from build123d import *

# Parameters (mm, degrees)
MODEL_R                 = 17.5
MODEL_R_2               = 1.5
SALIENTE_EXTRUIR1_DEPTH = 3


with BuildPart() as part:
    # Model → Saliente-Extruir1 (new body)
    with BuildSketch(Plane.XY):
        with BuildLine():
            Line((119.290027295, 223.651688958), (119.290027295, 219.036053988))
            Line((119.290027295, 219.036053988), (123.790027295, 219.036053988))
            Line((123.790027295, 219.036053988), (123.790027295, 210.036053988))
            Line((123.790027295, 210.036053988), (119.290027295, 210.036053988))
            Line((119.290027295, 210.036053988), (119.290027295, 183.036053988))
            Line((119.290027295, 183.036053988), (141.790027295, 183.036053988))
            Line((141.790027295, 183.036053988), (141.790027295, 192.036053988))
            Line((141.790027295, 192.036053988), (150.790027295, 192.036053988))
            Line((150.790027295, 192.036053988), (150.790027295, 183.036053988))
            Line((150.790027295, 183.036053988), (173.290027295, 183.036053988))
            Line((173.290027295, 183.036053988), (173.290027295, 210.036053988))
            Line((173.290027295, 210.036053988), (168.790027295, 210.036053988))
            Line((168.790027295, 210.036053988), (168.790027295, 219.036053988))
            Line((168.790027295, 219.036053988), (173.290027295, 219.036053988))
            Line((173.290027295, 219.036053988), (173.290027295, 223.651688958))
            Line((173.290027295, 223.651688958), (166.290027295, 229.536053988))
            ThreePointArc((166.290027295, 229.536053988), (164.825561201, 233.071587894), (161.290027295, 234.536053988))
            Line((161.290027295, 234.536053988), (131.290027295, 234.536053988))
            ThreePointArc((131.290027295, 234.536053988), (127.754493389, 233.071587894), (126.290027295, 229.536053988))
            Line((126.290027295, 229.536053988), (119.290027295, 223.651688958))
        make_face()
        with Locations((146.290027295, 214.536053988)):
            Circle(MODEL_R, mode=Mode.SUBTRACT)
        with Locations((168.790027295, 223.536053988)):
            Circle(MODEL_R_2, mode=Mode.SUBTRACT)
        with Locations((161.290027295, 229.536053988)):
            Circle(MODEL_R_2, mode=Mode.SUBTRACT)
        with Locations((168.790027295, 187.536053988)):
            Circle(MODEL_R_2, mode=Mode.SUBTRACT)
        with Locations((161.290027295, 199.536053988)):
            Circle(MODEL_R_2, mode=Mode.SUBTRACT)
        with Locations((123.790027295, 223.536053988)):
            Circle(MODEL_R_2, mode=Mode.SUBTRACT)
        with Locations((131.290027295, 229.536053988)):
            Circle(MODEL_R_2, mode=Mode.SUBTRACT)
        with Locations((131.290027295, 199.536053988)):
            Circle(MODEL_R_2, mode=Mode.SUBTRACT)
        with Locations((123.790027295, 187.536053988)):
            Circle(MODEL_R_2, mode=Mode.SUBTRACT)
        with BuildLine():
            Line((122.290027295, 203.286053988), (122.290027295, 198.786053988))
            ThreePointArc((122.290027295, 198.786053988), (123.790027295, 197.286053988), (125.290027295, 198.786053988))
            Line((125.290027295, 198.786053988), (125.290027295, 203.286053988))
            ThreePointArc((125.290027295, 203.286053988), (123.790027295, 204.786053988), (122.290027295, 203.286053988))
        make_face(mode=Mode.SUBTRACT)
        with BuildLine():
            Line((167.290027295, 203.286053988), (167.290027295, 198.786053988))
            ThreePointArc((167.290027295, 198.786053988), (168.790027295, 197.286053988), (170.290027295, 198.786053988))
            Line((170.290027295, 198.786053988), (170.290027295, 203.286053988))
            ThreePointArc((170.290027295, 203.286053988), (168.790027295, 204.786053988), (167.290027295, 203.286053988))
        make_face(mode=Mode.SUBTRACT)
        with BuildLine():
            Line((162.040027295, 189.036053988), (157.540027295, 189.036053988))
            ThreePointArc((157.540027295, 189.036053988), (156.040027295, 187.536053988), (157.540027295, 186.036053988))
            Line((157.540027295, 186.036053988), (162.040027295, 186.036053988))
            ThreePointArc((162.040027295, 186.036053988), (163.540027295, 187.536053988), (162.040027295, 189.036053988))
        make_face(mode=Mode.SUBTRACT)
        with BuildLine():
            Line((135.040027295, 186.036053988), (130.540027295, 186.036053988))
            ThreePointArc((130.540027295, 186.036053988), (129.040027295, 187.536053988), (130.540027295, 189.036053988))
            Line((130.540027295, 189.036053988), (135.040027295, 189.036053988))
            ThreePointArc((135.040027295, 189.036053988), (136.540027295, 187.536053988), (135.040027295, 186.036053988))
        make_face(mode=Mode.SUBTRACT)
    extrude(amount=SALIENTE_EXTRUIR1_DEPTH)


solid = part.part
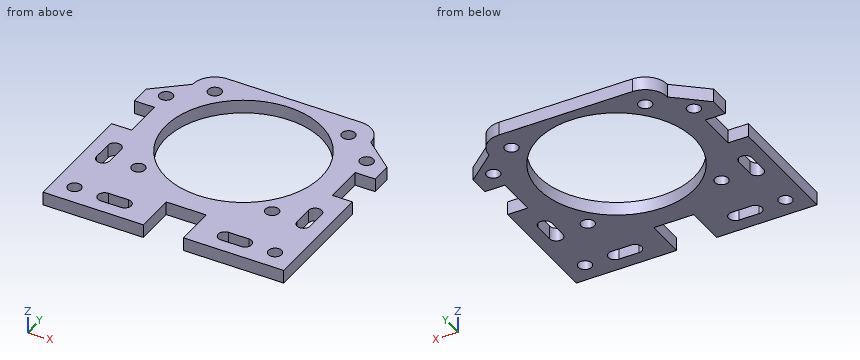
The listing builds one solid part. Answer for the finished solid, in the listing's coordinates (mm). Give positions to 0.01 mm unless a question says otherwise; leave off trailing zeros. Loops run counter-clockwise (first coordinate to the right, second up) from the corner with the lowest first, then second, coordinate; pieces in that order, holes last. Notation, with made-up numbers: (-32, 69) - (5, 69) arc R30 ccw to (5, 95) - close; hole circle Ø6 at (82, 58.25). An arc over 180 degrees is marked (long way). Use one line per item in the form item = value.
1. Given pin 1 Ø1 at (x, y) = (152.5, 229) entering from +Z, flat-ended and moving along its own axis, determine where the tip first touches the part or whether it passes through.
Calculated:
pin_1 = through
2. Find the intervals of material crossed by line 1 along X through (y, z) = (200, 1.8); line 2 along X through (y, z) = (185, 0.55); line 3 along Y through (x, z) = (125, 2.35), in increasing order. Write a range as [from, to].
Calculated:
line_1 = [119.29, 122.29], [125.29, 129.86], [132.72, 136.55], [156.03, 159.86], [162.72, 167.29], [170.29, 173.29]
line_2 = [119.29, 141.79], [150.79, 173.29]
line_3 = [183.04, 186.65], [188.42, 197.9], [204.17, 222.65], [224.42, 228.45]
3. Section D-D on z = 2.4 is taken. Count the separate pieces of the cut face and the enclosed holes in it, then the cut area to 3 significant figures.
Calculated:
separate_pieces = 1
enclosed_holes = 13
area = 1,400 mm^2
4. Section A-A on y = 191 is taken. Give the vertices of the cut face in (x, z).
Calculated:
outline = (119.29, 0) - (141.79, 0) - (141.79, 3) - (119.29, 3) - close; (150.79, 0) - (173.29, 0) - (173.29, 3) - (150.79, 3) - close
5. Section C-C on y = 204 is taken. Give the vertices of the cut face in (x, z).
Calculated:
outline = (119.29, 0) - (122.47, 0) - (122.47, 3) - (119.29, 3) - close; (125.11, 0) - (132.32, 0) - (132.32, 3) - (125.11, 3) - close; (160.26, 0) - (167.47, 0) - (167.47, 3) - (160.26, 3) - close; (170.11, 0) - (173.29, 0) - (173.29, 3) - (170.11, 3) - close
6. Section B-B on x = 152 is taken. Give the vertices of the cut face in (y, z), then the cut area to 3 significant figures.
Calculated:
outline = (183.04, 0) - (197.99, 0) - (197.99, 3) - (183.04, 3) - close; (231.08, 0) - (234.54, 0) - (234.54, 3) - (231.08, 3) - close
area = 55.2 mm^2
